CAD build for the part. Positions are in the model's coordinates, mm. A direction names the side the tool comes from. Give positions to 0.01 mm unless a question says otherwise; leave off trailing zeros. Loops run counter-clockwise (first coordinate to the right, second up) from the corner with the lowest first, then second, coordinate; pieces in that order, holes last.
```python
from build123d import *

# Parameters (mm, degrees)
BOSS_EXTRUDE1_DEPTH        = 6.35
BOSS_EXTRUDE1_DEPTH_BACK   = 6.35
BOSS_EXTRUDE1_2_DEPTH      = 6.35
BOSS_EXTRUDE1_2_DEPTH_BACK = 6.35
BOSS_EXTRUDE2_DEPTH        = 6.35
BOSS_EXTRUDE2_DEPTH_BACK   = 6.35
SKETCH3_W                  = 0.4572
SKETCH3_H                  = 44.508
BOSS_EXTRUDE4_DEPTH        = 6.35
BOSS_EXTRUDE4_DEPTH_BACK   = 6.35
SKETCH8_W                  = 2.032
SKETCH8_H                  = 1.778
CUT_EXTRUDE1_DEPTH         = 63.522062345
FILLET1_R                  = 0.4572
FILLET2_R                  = 0.9144
FILLET3_R                  = 3.556
FILLET6_R                  = 12.7
SKETCH9_R                  = 1.1303
CUT_EXTRUDE2_DEPTH         = 63.522062345
FILLET7_R                  = 0.127
FILLET8_R                  = 0.508
FILLET9_R                  = 76.2
SKETCH12_W                 = 3.975578287
SKETCH12_H                 = 4.68929279
SKETCH12_W_2               = 5.470600001
SKETCH12_H_2               = 8.387314833
CUT_EXTRUDE3_DEPTH         = 63.522062345
FILLET10_R                 = 0.127


with BuildPart() as part:
    # Sketch2 → Boss-Extrude1 (new, two sides: drawn at the far end of the back side and taken through both)
    with BuildSketch(Plane(origin=(0, 0, 0), x_dir=(1, 0, 0), z_dir=(0, 1, 0)).offset(-BOSS_EXTRUDE1_DEPTH_BACK)):
        with BuildLine():
            Line((9.819911786, 19.050210052), (19.344911786, 19.050210052))
            Line((19.344911786, 19.050210052), (21.965511899, 22))
            Line((21.965511899, 22), (24.251511899, 22))
            Line((24.251511899, 22), (29.687111899, -2.381342584))
            Line((29.687111899, -2.381342584), (35.584296061, -2.381342584))
            Line((35.584296061, -2.381342584), (50.68062, -7.62))
            Line((50.68062, -7.62), (50.68062, 7.62))
            Line((50.68062, 7.62), (35.584296061, 2.381342584))
            Line((35.584296061, 2.381342584), (28.784210924, 23.462125012))
            ThreePointArc((28.784210924, 23.462125012), (27.055039043, 25.850117603), (24.251511899, 26.762685167))
            Line((24.251511899, 26.762685167), (-6.638632099, 26.762685167))
            Line((-6.638632099, 26.762685167), (-30.153140375, 24.092168337))
            Line((-30.153140375, 24.092168337), (-42.245281802, 26.68929279))
            Line((-42.245281802, 26.68929279), (-48.211266614, 26.68929279))
            Line((-48.211266614, 26.68929279), (-48.211266614, 22))
            Line((-48.211266614, 22), (-38.957383068, 22))
            Line((-38.957383068, 22), (-36.496303445, 20.550210052))
            Line((-36.496303445, 20.550210052), (-1.229088214, 20.550210052))
            Line((-1.229088214, 20.550210052), (9.819911786, 19.050210052))
        make_face()
    extrude(amount=BOSS_EXTRUDE1_DEPTH + BOSS_EXTRUDE1_DEPTH_BACK)



with BuildPart() as body_2:
    # Sketch2 → Boss-Extrude1 2 (new, two sides: drawn at the far end of the back side and taken through both)
    with BuildSketch(Plane(origin=(0, 0, 0), x_dir=(1, 0, 0), z_dir=(0, 1, 0)).offset(-BOSS_EXTRUDE1_2_DEPTH_BACK)):
        Polygon((-50.68062, 7.62), (-47.994229245, 7.62), (-45.538273994, 0.064709726), (-44.235688327, -22), (-41.949688327, -22), (-39.329088214, -19.050210052), (-14.524057774, -19.050210052), (6.319911674, -20.5502101), (6.319911674, -24.799314833), (16.494911898, -24.799314833), (16.494911898, -22), (16.494911898, -20.7842203), (18.962447951, -22), (29.7221119, -22), (29.7221119, -24.341022744), (19.249626804, -30.387314833), (-1.624639293, -30.387314833), (-27.239820872, -25.774174137), (-37.984514025, -25.774174137), (-49.463347649, -28.239573642), (-50.68062, -7.62), align=None)
    extrude(amount=BOSS_EXTRUDE1_2_DEPTH + BOSS_EXTRUDE1_2_DEPTH_BACK)


with BuildPart() as part_1:
    add(part.part)

    add(body_2.part)  # Boss-Extrude2 merges body 2
    # Sketch3 → Boss-Extrude2 (add, two sides: drawn at the far end of the back side and taken through both)
    with BuildSketch(Plane(origin=(0, 0, 0), x_dir=(1, 0, 0), z_dir=(0, 1, 0)).offset(-BOSS_EXTRUDE2_DEPTH_BACK)):
        with Locations((-43.092688327, 0.254)):
            Rectangle(SKETCH3_W, SKETCH3_H)
        with Locations((23.108511899, 0.254)):
            Rectangle(SKETCH3_W, SKETCH3_H)
    extrude(amount=BOSS_EXTRUDE2_DEPTH + BOSS_EXTRUDE2_DEPTH_BACK)

    # Sketch7 → Boss-Extrude4 (add, two sides: drawn at the far end of the back side and taken through both)
    with BuildSketch(Plane(origin=(0, 0, 0), x_dir=(1, 0, 0), z_dir=(0, 1, 0)).offset(-BOSS_EXTRUDE4_DEPTH_BACK)):
        Polygon((-53.14442, 3.68670581), (-53.14442, -3.68670581), (-50.75682, -2.49290581), (-50.68062, -2.45480581), (-50.68062, 2.45480581), (-50.75682, 2.49290581), align=None)
        Polygon((50.68062, 2.45480581), (50.68062, -2.45480581), (50.75682, -2.49290581), (53.14442, -3.68670581), (53.14442, 3.68670581), (50.75682, 2.49290581), align=None)
    extrude(amount=BOSS_EXTRUDE4_DEPTH + BOSS_EXTRUDE4_DEPTH_BACK)

    # Sketch8 → Cut-Extrude1 (cut, through all)
    with BuildSketch(Plane(origin=(0, 6.35, 0), x_dir=(1, 0, 0), z_dir=(0, 1, 0))):
        with Locations((-52.25542, 0)):
            Rectangle(SKETCH8_W, SKETCH8_H)
        with Locations((52.25542, 0)):
            Rectangle(SKETCH8_W, SKETCH8_H)
    extrude(amount=-CUT_EXTRUDE1_DEPTH, mode=Mode.SUBTRACT)

    # Fillet1
    fillet1_edges = [part_1.edges().sort_by_distance(p)[0] for p in [
        (-43.321288327, 0, -22),
        (24.251511899, 0, -22),
        (21.965511899, 0, -22),
        (-42.864088327, 0, -22),
        (23.337111899, 0, -22),
        (22.879911899, 0, -22),
        (22.879911899, 0, 22),
        (23.337111899, 0, 22),
        (-44.235688327, 0, 22),
        (-41.949688327, 0, 22),
        (-42.864088327, 0, 22),
        (-43.321288327, 0, 22),
    ]]
    fillet(fillet1_edges, radius=FILLET1_R)

    # Fillet2
    fillet2_edges = [part_1.edges().sort_by_distance(p)[0] for p in [
        (29.687111899, 0, 2.381342584),
        (-48.211266614, 0, -22),
        (-48.211266614, 0, -26.68929279),
        (29.7221119, 0, 22),
        (29.7221119, 0, 24.341022744),
    ]]
    fillet(fillet2_edges, radius=FILLET2_R)

    # Fillet3
    fillet3_edges = [part_1.edges().sort_by_distance(p)[0] for p in [
        (35.584296061, 0, -2.381342584),
        (19.249626804, 0, 30.387314833),
        (-49.463347649, 0, 28.239573642),
    ]]
    fillet(fillet3_edges, radius=FILLET3_R)

    # Fillet6
    # the kernel refuses this fillet: 12.7 mm, written as the material it adds along each edge
    with BuildSketch(Plane(origin=(-37.984514025, 6.35, 25.774174137), x_dir=(1, 0, 0), z_dir=(0, -1, 0))) as fillet6_piece_1:
        with BuildLine():
            CenterArc((FILLET6_R * 0.106178254311, FILLET6_R), FILLET6_R, 257.878284844, 12.121715156)
            Line((-FILLET6_R * 0.103810874318, FILLET6_R * 0.0222962791022), (0, 0))
            Line((0, 0), (FILLET6_R * 0.106178254311, 0))
        make_face()
    extrude(amount=12.7)
    # the kernel refuses this fillet: 12.7 mm, written as the material it takes off along each edge
    with BuildSketch(Plane(origin=(-36.496303445, 14.928809219, -20.550210052), x_dir=(-0.8616133508003352, 0, -0.507565201449645), z_dir=(0, -1, 0))) as fillet6_2_piece_1:
        with BuildLine():
            CenterArc((3.489431436, 12.684211567), FILLET6_R, 239.498215304, 27.644521231)
            Line((-2.956646623, 1.741722012), (0, 0))
            Line((0, 0), (2.856361988, 0))
        make_face()
    extrude(amount=29.857618438, mode=Mode.SUBTRACT)

    # Sketch9 → Cut-Extrude2 (cut, through all)
    with BuildSketch(Plane(origin=(0, 6.35, 0), x_dir=(1, 0, 0), z_dir=(0, 1, 0))):
        with Locations(Location((-37.678088214, -22.225210052, 0), (0, 0, 270))):
            Circle(SKETCH9_R)
        with Locations(Location((-32.598088214, -22.225210052, 0), (0, 0, 270))):
            Circle(SKETCH9_R)
        with Locations(Location((12.613911786, 22.225210052, 0), (0, 0, 270))):
            Circle(SKETCH9_R)
        with Locations(Location((17.693911786, 22.225210052, 0), (0, 0, 270))):
            Circle(SKETCH9_R)
    extrude(amount=-CUT_EXTRUDE2_DEPTH, mode=Mode.SUBTRACT)

    # Fillet7
    fillet7_edges = [part_1.edges().sort_by_distance(p)[0] for p in [
        (16.494911898, 0, 20.7842203),
    ]]
    fillet(fillet7_edges, radius=FILLET7_R)

    # Fillet8
    fillet8_edges = [part_1.edges().sort_by_distance(p)[0] for p in [
        (6.319911674, 0, 24.799314833),
        (16.494911898, 0, 24.799314833),
    ]]
    fillet(fillet8_edges, radius=FILLET8_R)

    # Fillet9
    # the kernel refuses this fillet: 76.2 mm, written as the material it adds along each edge
    with BuildSketch(Plane(origin=(-30.153140375, -6.35, -24.092168337), x_dir=(-0.9777037208978189, 0, -0.20998912862945954), z_dir=(0, 1, 0))) as fillet9_piece_1_section:
        with BuildLine():
            CenterArc((FILLET9_R * 0.16376499609, -FILLET9_R), FILLET9_R, 90, 18.600972695)
            Line((-FILLET9_R * 0.155210403169, -FILLET9_R * 0.0522370050125), (0, 0))
            Line((0, 0), (FILLET9_R * 0.16376499609, 0))
        make_face()
    fillet9_piece_1 = extrude(amount=12.7, mode=Mode.PRIVATE)
    fillet9_piece_1 = split(fillet9_piece_1, bisect_by=Plane(origin=(-30.153140375, -6.35, -26.68929279), z_dir=(0, 0, 1)), keep=Keep.TOP, mode=Mode.PRIVATE)
    add(fillet9_piece_1)

    # Sketch12 → Cut-Extrude3 (cut, through all)
    with BuildSketch(Plane(origin=(0, 6.35, 0), x_dir=(1, 0, 0), z_dir=(0, 1, 0))):
        with Locations((-46.223477471, 24.344646395)):
            Rectangle(SKETCH12_W, SKETCH12_H)
        with Locations((26.9868119, -26.193657417)):
            Rectangle(SKETCH12_W_2, SKETCH12_H_2)
    extrude(amount=-CUT_EXTRUDE3_DEPTH, mode=Mode.SUBTRACT)

    # Fillet10
    fillet10_edges = [part_1.edges().sort_by_distance(p)[0] for p in [
        (50.68062, 0, -2.45480581),
        (50.68062, 0, 2.45480581),
        (53.14442, 0, 3.68670581),
        (53.14442, 0, -3.68670581),
        (-50.68062, 0, 2.45480581),
        (-50.68062, 0, -2.45480581),
        (-53.14442, 0, -3.68670581),
        (-53.14442, 0, 3.68670581),
    ]]
    fillet(fillet10_edges, radius=FILLET10_R)


solid = part_1.part
```
1. Pull direction X, two halves, no side cores. Call faces 4 (the face through (-53.144, 0, 2)), 5 (the face through (-4.25, -0.09, 19.79)), 6 (the face through (53.144, 0, 2)): released by +X, released by -X, zero draft, split by the parting line, or undercut.
Responses:
face 4: released by -X
face 5: undercut
face 6: released by +X
2. Saw through at C-C, the plane z = 5.5. List the corners of the cut face in (x, y), and give its area (3 significant figures).
Responses:
outline: (-50.68, -6.35) - (-45.21, -6.35) - (-45.21, 6.35) - (-50.68, 6.35) - close; (-43.32, -6.35) - (-42.86, -6.35) - (-42.86, 6.35) - (-43.32, 6.35) - close; (22.88, -6.35) - (23.34, -6.35) - (23.34, 6.35) - (22.88, 6.35) - close; (44.57, -6.35) - (50.68, -6.35) - (50.68, 6.35) - (44.57, 6.35) - close
area: 159 mm2
3. Saw through at B-B, the plane z = 11.5. List the corners of the cut face in (x, y).
Responses:
outline: (-50.45, -6.35) - (-44.86, -6.35) - (-44.86, 6.35) - (-50.45, 6.35) - close; (-43.32, -6.35) - (-42.86, -6.35) - (-42.86, 6.35) - (-43.32, 6.35) - close; (22.88, -6.35) - (23.34, -6.35) - (23.34, 6.35) - (22.88, 6.35) - close
4. Saw through at D-D, the plane x = 2.5. List the corners of the cut face in (y, z).
Responses:
outline: (-6.35, -26.76) - (6.35, -26.76) - (6.35, -20.04) - (-6.35, -20.04) - close; (-6.35, 20.28) - (6.35, 20.28) - (6.35, 30.39) - (-6.35, 30.39) - close
5. Tool access for faces 1 (the face through (-27, 0, 19.05)), 2 (the face through (-32, 0, 25.774)), 3 (the face through (52, 0, 0.889)): list every direction of +Z, -Z, +X, -X, +Y, -Y with a clear straight run to the whole face (end or side of a thin tool).
Responses:
face 1: +Y, -Y
face 2: +Z, +Y, -Y
face 3: +X, +Y, -Y
6. Saw through at A-A, the plane x = -20.5. List the corners of the cut face in (y, z).
Responses:
outline: (-6.35, -25.24) - (6.35, -25.24) - (6.35, -20.55) - (-6.35, -20.55) - close; (-6.35, 19.05) - (6.35, 19.05) - (6.35, 26.99) - (-6.35, 26.99) - close
7. Drop flat-ended pins along their axis: pin 1 (1 mm diameter, centred on x = -28.5, y = 0, fed in from -Z); pin 2 (0.5 mm diameter, centred on x = -44, y = 2.5, fed in from +Z); pin 3 (5 mm diameter, centred on y = -4.5, z = 4.5, fed in from -X); pin 4 (1 mm diameter, centred on x = -43.5, y = 0, fed in from -Z). Give the stop position or say it passes through.
Responses:
pin 1: stops at z = -25.06
pin 2: stops at z = 27.12
pin 3: stops at x = -53.14
pin 4: stops at z = -26.69
8. Probe line 1 along X through (y, z) = (0.75, -12); line 2 along X through (y, z) = (-3, -17); line 3 along Z through (x, y) = (-16, 4.5). List the from-to ranges inside material, lowest first.
Responses:
line 1: x = -43.32 to -42.86, 22.88 to 23.34, 26.48 to 32.48
line 2: x = -43.32 to -42.86, 22.88 to 23.34, 25.37 to 30.87
line 3: z = -25.7 to -20.55, 19.05 to 27.8
